```python
from build123d import *

# Parameters (mm, degrees)
SKETCH1_W           = 30.2
SKETCH1_H           = 30.2
SKETCH1_W_2         = 20.2
SKETCH1_H_2         = 20.2
EXTRUDE_THIN1_DEPTH = 30
SKETCH2_R           = 4
BOSS_EXTRUDE1_DEPTH = 30.2
FILLET1_R           = 10


with BuildPart() as part:
    # Sketch1 → Extrude-Thin1 (new body)
    with BuildSketch(Plane(origin=(0, 0, 0), x_dir=(1, 0, 0), z_dir=(0, 1, 0))):
        with Locations((10.1, 10.1)):
            Rectangle(SKETCH1_W, SKETCH1_H)
        with Locations((10.1, 10.1)):
            Rectangle(SKETCH1_W_2, SKETCH1_H_2, mode=Mode.SUBTRACT)
    extrude(amount=EXTRUDE_THIN1_DEPTH)

    # Sketch2 → Boss-Extrude1 (add)
    with BuildSketch(Plane.XY.offset(5)):
        with BuildLine():
            Line((37.472155728, 20.545149722), (25.2, 30))
            Line((25.2, 30), (25.2, 0))
            Line((25.2, 0), (37.472155728, 9.454850278))
            ThreePointArc((37.472155728, 9.454850278), (40.2, 15), (37.472155728, 20.545149722))
        make_face()
        with Locations((33.2, 15)):
            Circle(SKETCH2_R, mode=Mode.SUBTRACT)
    extrude(amount=-BOSS_EXTRUDE1_DEPTH)

    # Fillet1
    fillet1_edges = [part.edges().sort_by_distance(p)[0] for p in [
        (25.2, 30, -10.1),
        (25.2, 0, -10.1),
    ]]
    fillet(fillet1_edges, radius=FILLET1_R)


solid = part.part
```
The listing builds one solid part. Answer for the finished solid, in the listing's coordinates (mm). A direction names the side the tool comes from. Give positions to 0.01 mm unless a question says otherwise; leave off trailing zeros. Order: outer loops, then holes, each group sorted by start corner. A loop starts at its lowest first (then second) coordinate and runs counter-clockwise, first axis right, second up. Notation, with made-up numbers: M -18,-21 L 32,-21 A23 ccw 32,13 Z; hole C -4.5,-30 d1. An arc over 180 degrees is marked long. Put each result on its own line as item: value. Start each with the question number.
Item 1: The part is cut by section D-D, the plane z = -23. Determine the outline of the cut face in (x, y), and give its area (3 significant figures).
Item 2: For a pull along X with two mould halves and no side action, classify faces 1 (the face through (37.015, 16.201, -9.889)), 2 (the face through (32.6, 5.7, -9.9)), 3 (the face through (-1, 0, -14)) as +X half, -X half, draft (parallel to the pull), parting line (faces both ways), or undercut.
Item 3: The part is cut by section C-C, the plane x = 9. Determine the outline of the cut face in (y, z), and give its area (3 significant figures).
Item 4: Which of the six approach directions +Z, -Z, +X, -X, +Y, -Y give full straight-line access (tool end or side, diameter ignored) to faces 4 (the face through (-5, 15, -10)), 5 (the face through (10, 15, -20.2))?
Item 5: Flat-ended cylindrical pins translate along their axes: P1, Ø10, axis at y = 26, z = -12, coming from the +X side; P2, Ø10, axis at y = 21, z = -12, coming from the +X side. Find the tip coordinate at first contact, or state that the pin passes through.
Item 6: The part is cut by section A-A, the plane z = -15.5. Determine the outline of the cut face in (x, y), and give its area (3 significant figures).
Item 7: The part is cut by section B-B, the plane y = 15. Determine the outline of the cut face in (x, z), and give its area (3 significant figures).
Item 8: Find the intervals of material crossed by line 1 along X through (y, z) = (14.75, -9); line 2 along Z through (x, y) = (9.5, 16.5); line 3 along Y through (x, z) = (31, -5), in increasing order.
Answer key:
1. outline: M -5,0 L 21.79,0 A10 ccw 27.9,2.08 L 37.47,9.45 A7 ccw 37.47,20.55 L 27.9,27.92 A10 ccw 21.79,30 L -5,30 Z; hole C 33.2,15 d8
1. area: 1,130 mm²
2. face 1: undercut
2. face 2: +X half
2. face 3: draft
3. outline: M 0,-25.2 L 30,-25.2 L 30,-20.2 L 0,-20.2 Z; M 0,0 L 30,0 L 30,5 L 0,5 Z
3. area: 300 mm²
4. face 4: +Z, -Z, -X, +Y, -Y
4. face 5: +Y, -Y
5. P1: stops at x = 36.88
5. P2: stops at x = 40.13
6. outline: M -5,0 L 0,0 L 0,30 L -5,30 Z; M 20.2,0 L 21.79,0 A10 ccw 27.9,2.08 L 37.47,9.45 A7 ccw 37.47,20.55 L 27.9,27.92 A10 ccw 21.79,30 L 20.2,30 Z; hole C 33.2,15 d8
6. area: 521 mm²
7. outline: M -5,-25.2 L 29.2,-25.2 L 29.2,5 L -5,5 Z; M 37.2,-25.2 L 40.2,-25.2 L 40.2,5 L 37.2,5 Z; hole M 0,-20.2 L 20.2,-20.2 L 20.2,0 L 0,0 Z
7. area: 715 mm²
8. line 1: x = -5 to 0, 20.2 to 29.21, 37.19 to 40.2
8. line 2: z = -25.2 to -20.2, 0 to 5
8. line 3: y = 4.47 to 11.66, 18.34 to 25.53
